from build123d import *

# Parameters (mm, degrees)
ESQUISSE2_W                                       = 80
ESQUISSE2_H                                       = 85
PLAQUE_DEPTH                                      = 5.4
ESQUISSE15_R                                      = 22
D_GAGEMENT_ROUE_DEPTH                             = 81.678373806
D_COUPE_INF_RIEURE_DEPTH                          = 81.803217758
ESQUISSE14_R                                      = 11.05
ESQUISSE14_R_2                                    = 5.05
RENFORT_ROULEMENT_DEPTH                           = 2.4
D_COUPE_SUP_RIEURE_DEPTH                          = 81.803217758
D_GAGEMENT_AXE_6_DEPTH                            = 75.400336021
D_GAGEMENT_AXE_6_DEPTH_BACK                       = 75.400336021
ESQUISSE26_W                                      = 6.8
ESQUISSE26_H                                      = 6.8
D_GAGEMENT_START                                  = 1.4
D_GAGEMENT_DOUILLE_DEPTH                          = 19.2
R_P_TITION_LIN_AIRE1_COUNT                        = 2
R_P_TITION_LIN_AIRE1_PITCH                        = 26
MORS_D_FORMABLE_DOUILLE_DEPTH                     = 75.400336021
MORS_D_FORMABLE_DOUILLE_DEPTH_BACK                = 75.400336021
FRAISAGE_POUR_VIS_T_TE_FRAIS_E_BOMB_E_D           = 3.2
FRAISAGE_POUR_VIS_T_TE_FRAIS_E_BOMB_E_CSINK_D     = 6.92
FRAISAGE_POUR_VIS_T_TE_FRAIS_E_BOMB_E_CSINK_ANGLE = 90
ESQUISSE31_W                                      = 80
ESQUISSE31_H                                      = 35.1
ENL_V_MAT_EXTRU_1_DEPTH                           = 5.4
BOSS_EXTRU_1_DEPTH                                = 2.4
ESQUISSE34_R                                      = 1.55
ENL_V_MAT_EXTRU_2_DEPTH                           = 10


with BuildPart() as part:
    # Esquisse2 → plaque (new body)
    with BuildSketch(Plane(origin=(0, 0, 0), x_dir=(0, 0, -1), z_dir=(1, 0, 0))):
        with Locations((0, 27.5)):
            Rectangle(ESQUISSE2_W, ESQUISSE2_H)
    extrude(amount=PLAQUE_DEPTH)

    # Esquisse15 → dégagement roue (cut, through all)
    with BuildSketch(Plane.ZY.offset(-2.4)):
        with Locations((0, -12)):
            Circle(ESQUISSE15_R)
    extrude(amount=-D_GAGEMENT_ROUE_DEPTH, mode=Mode.SUBTRACT)

    # Esquisse18 → découpe_inférieure (cut, through all)
    with BuildSketch(Plane(origin=(0, 0, 0), x_dir=(0, 0, -1), z_dir=(1, 0, 0))):
        Polygon((-7.446869682, -5.5), (-40, -5.5), (-40, -15), (40, -15), (40, -5.5), (7.446869682, -5.5), align=None)
    extrude(amount=D_COUPE_INF_RIEURE_DEPTH, mode=Mode.SUBTRACT)

    # Esquisse14 → renfort_roulement (add)
    with BuildSketch(Plane(origin=(0, 0, 0), x_dir=(0, 0, -1), z_dir=(1, 0, 0))):
        with Locations((0, -12)):
            Circle(ESQUISSE14_R)
        with Locations((0, -12)):
            Circle(ESQUISSE14_R_2, mode=Mode.SUBTRACT)
    extrude(amount=RENFORT_ROULEMENT_DEPTH)

    # Esquisse20 → découpe_supérieure (cut, through all)
    with BuildSketch(Plane(origin=(0, 0, 0), x_dir=(0, 0, -1), z_dir=(1, 0, 0))):
        with BuildLine():
            Line((-40, 70), (40, 70))
            Line((40, 70), (40, 62.5))
            Line((40, 62.5), (26, 62.5))
            ThreePointArc((26, 62.5), (22.956192855, 61.466766701), (21.170370869, 58.794095226))
            Line((21.170370869, 58.794095226), (15.559208556, 37.852952387))
            ThreePointArc((15.559208556, 37.852952387), (14.666297563, 36.516616649), (13.144393991, 36))
            Line((13.144393991, 36), (-13.144393991, 36))
            ThreePointArc((-13.144393991, 36), (-14.666297563, 36.516616649), (-15.559208556, 37.852952387))
            Line((-15.559208556, 37.852952387), (-21.170370869, 58.794095226))
            ThreePointArc((-21.170370869, 58.794095226), (-22.956192855, 61.466766701), (-26, 62.5))
            Line((-26, 62.5), (-40, 62.5))
            Line((-40, 62.5), (-40, 70))
        make_face()
    extrude(amount=D_COUPE_SUP_RIEURE_DEPTH, mode=Mode.SUBTRACT)

    # Esquisse26 → dégagement axe 6 (cut, two sides: drawn at the far end of the back side and taken through both)
    with BuildSketch(Plane(origin=(0, 0, 0), x_dir=(1, 0, 0), z_dir=(0, 1, 0)).offset(-D_GAGEMENT_AXE_6_DEPTH_BACK)):
        with Locations((5.9, 31.5)):
            Rectangle(ESQUISSE26_W, ESQUISSE26_H)
        with Locations((5.9, -31.5)):
            Rectangle(ESQUISSE26_W, ESQUISSE26_H)
    extrude(amount=D_GAGEMENT_AXE_6_DEPTH + D_GAGEMENT_AXE_6_DEPTH_BACK, mode=Mode.SUBTRACT)

    # Esquisse28 → dégagement douille (cut)
    with BuildSketch(Plane(origin=(0, 0, 0), x_dir=(1, 0, 0), z_dir=(0, 1, 0)).offset(D_GAGEMENT_START)):
        Polygon((0, 35.5), (1.427864045, 35.5), (1.427864045, 37.7), (10.372135955, 37.7), (10.372135955, 25.3), (1.427864045, 25.3), (1.427864045, 27.5), (0, 27.5), align=None)
        Polygon((10.372135955, -25.3), (1.427864045, -25.3), (1.427864045, -27.5), (0, -27.5), (0, -35.5), (1.427864045, -35.5), (1.427864045, -37.7), (10.372135955, -37.7), align=None)
    d_gagement_douille = extrude(amount=D_GAGEMENT_DOUILLE_DEPTH, mode=Mode.SUBTRACT)

    # Répétition linéaire1: dégagement douille ×2
    with Locations(*[(0, i * R_P_TITION_LIN_AIRE1_PITCH, 0) for i in range(1, R_P_TITION_LIN_AIRE1_COUNT)]):
        add(d_gagement_douille, mode=Mode.SUBTRACT)

    # Esquisse19 → Mors_déformable_douille (cut, two sides: drawn at the far end of the back side and taken through both)
    with BuildSketch(Plane(origin=(0, 0, 0), x_dir=(1, 0, 0), z_dir=(0, 1, 0)).offset(-MORS_D_FORMABLE_DOUILLE_DEPTH_BACK)):
        Polygon((5.4, 40), (4.4, 40), (4.4, 24.1), (1, 24.1), (1, 23), (5.4, 23), align=None)
    extrude(amount=MORS_D_FORMABLE_DOUILLE_DEPTH + MORS_D_FORMABLE_DOUILLE_DEPTH_BACK, mode=Mode.SUBTRACT)

    # Fraisage pour vis à tête fraisée bombée fendue M31 (through all)
    with Locations(Plane.ZY):
        with Locations((18, 18), (36.7, 24), (36.7, -2), (21, 34)):
            fraisage_pour_vis_t_te_frais_e_bomb_e = CounterSinkHole(FRAISAGE_POUR_VIS_T_TE_FRAIS_E_BOMB_E_D / 2, FRAISAGE_POUR_VIS_T_TE_FRAIS_E_BOMB_E_CSINK_D / 2, counter_sink_angle=FRAISAGE_POUR_VIS_T_TE_FRAIS_E_BOMB_E_CSINK_ANGLE)

    # Esquisse31 → Enlèv. mat.-Extru.1 (cut)
    with BuildSketch(Plane(origin=(5.4, 0, 0), x_dir=(0, 0, -1), z_dir=(1, 0, 0))):
        with Locations((0, 44.95)):
            Rectangle(ESQUISSE31_W, ESQUISSE31_H)
    extrude(amount=-ENL_V_MAT_EXTRU_1_DEPTH, mode=Mode.SUBTRACT)

    # Esquisse33 → Boss.-Extru.1 (add)
    with BuildSketch(Plane(origin=(2.4, 0, 0), x_dir=(0, 0, -1), z_dir=(1, 0, 0))):
        Polygon((-8.125418007, -19.488663579), (-21.017849557, -5.5), (-8.936022605, -5.5), align=None)
        Polygon((8.125418007, -19.488663579), (21.017849557, -5.5), (8.936022605, -5.5), align=None)
    extrude(amount=-BOSS_EXTRU_1_DEPTH)

    # Symétrie4: Fraisage pour vis à tête fraisée bombée fendue M31 across plane
    add(fraisage_pour_vis_t_te_frais_e_bomb_e.mirror(Plane.XY), mode=Mode.SUBTRACT)

    # Esquisse34 → Enlèv. mat.-Extru.2 (cut)
    with BuildSketch(Plane(origin=(2.4, 0, 0), x_dir=(0, 0, -1), z_dir=(1, 0, 0))):
        with Locations((-10.48, 3.75)):
            Circle(ESQUISSE34_R)
        with Locations((10.48, 3.75)):
            Circle(ESQUISSE34_R)
    extrude(amount=-ENL_V_MAT_EXTRU_2_DEPTH, mode=Mode.SUBTRACT)


solid = part.part
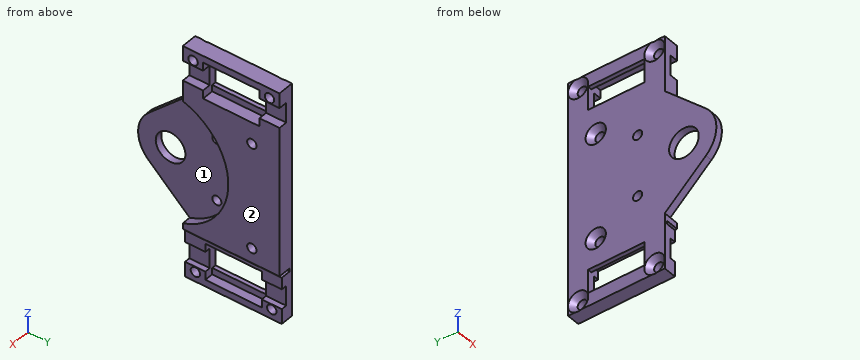
Geometry check sheet. Reference: the model listing, model coordinates, mm. Face numbers are marked on the shaded views. Coordinates: 2 decimals unless noted, no trailing zeros. Order: outer loops, then holes, each group sorted by start corner. A loop starts at its lowest first (then second) coordinate and runs counter-clockwise, first axis right, second up. Notation, with made-up numbers: (-39.75, 1.5) - (-14.75, 1.5) arc R8 cw to (-14.75, 12.5) - close; hole circle Ø1 at (-26, 42.25). An arc over 180 degrees is marked (long way). Answer in a Markdown table with one row per item. Add a question column.
1) Cross-section at C-C, the plane y = -12. Record the cut outline in (x, z).
2) Release check for a two-part mould opening along Z. For the marked faces 1 and 2 record: +Z half, -Z half, draft (parallel to the pull), parting line (faces both ways), or undercut.
3) Material ranges on line 1 along Z through (x, y) = (3.9, 24); line 2 along Z through (x, y) = (0.3, 11); line 3 along Y through (x, z) = (3.7, -36.7), recorded low to high. Write a range as [from, to].
4) Cross-section at B-B, the plane y = 24. Record the cut outline in (x, z).
5) Cross-section at A-A, the plane z = 29. Record the cut outline in (x, y).
6) Gauge pin test, flat ends, axial feed: P1, Ø5.5, axis at y = 5, z = -38.5, coming from the +X side; P2, Ø5, axis at y = 3.75, z = -10.48, coming from the +X side; P3, Ø2, axis at y = 24, z = -31.5, coming from the +X side. Record the tip position at first contact, or that the pin passes through.
7) Cross-section at D-D, the plane z = 0. Record the cut outline in (x, y), then the cut area to 3 significant figures.
Check result:
| question | item | result |
|---|---|---|
| 1 | outline | (0, -15.03) - (2.4, -15.03) - (2.4, -5.05) - (0, -5.05) - close; (0, 5.05) - (2.4, 5.05) - (2.4, 15.03) - (0, 15.03) - close |
| 2 | face 1 | undercut |
| 2 | face 2 | draft |
| 3 | line 1 | z = [-40, -38.3], [-35.1, -34.9], [-28.1, -24.1], [-23, 28.1], [34.9, 35.1], [38.3, 40] |
| 3 | line 2 | z = [-40, -35.5], [-27.5, 27.5], [35.5, 40] |
| 3 | line 3 | y = [-5.5, -3.6], [-0.4, 1.4], [20.6, 22.4], [25.6, 27.4] |
| 4 | outline | (0, -33.24) - (1.86, -35.1) - (4.4, -35.1) - (4.4, -34.9) - (2.5, -34.9) - (2.5, -28.1) - (4.4, -28.1) - (4.4, -24.1) - (1, -24.1) - (1, -23) - (5.4, -23) - (5.4, 28.1) - (2.5, 28.1) - (2.5, 34.9) - (5.4, 34.9) - (5.4, 35.1) - (1.86, 35.1) - (0, 33.24) - close; (0.16, -40) - (4.4, -40) - (4.4, -38.3) - (1.86, -38.3) - close; (0.16, 40) - (1.86, 38.3) - (5.4, 38.3) - (5.4, 40) - close |
| 5 | outline | (0, -5.5) - (2.5, -5.5) - (2.5, 1.4) - (0, 1.4) - close; (0, 20.6) - (2.5, 20.6) - (2.5, 27.4) - (0, 27.4) - close |
| 6 | P1 | stops at x = 4.4 |
| 6 | P2 | stops at x = 2.4 |
| 6 | P3 | stops at x = 2.5 |
| 7 | outline | (0, -23.05) - (2.4, -23.05) - (2.4, -17.05) - (0, -17.05) - close; (0, -6.95) - (2.4, -6.95) - (2.4, 10) - (5.4, 10) - (5.4, 27.4) - (0, 27.4) - close |
| 7 | area | 149 mm² |
